Autodesk Inventor part; units mm, degrees
ref_plane "YZ Plane" through (0, 0, 0) normal (1, 0, 0) x (0, 1, 0)
ref_plane "XZ Plane" through (0, 0, 0) normal (0, 1, 0) x (-1, 0, 0)
ref_plane "XY Plane" through (0, 0, 0) normal (0, 0, 1) x (1, 0, 0)
sketch "Sketch1" plane through (0, 0, 0) normal (0, 1, 0) x (-1, 0, 0)
  circle A0 centre (0, 0) radius 75
  circle A1 centre (0, 0) radius 63.5
  line L0 (62, 12.5) -> (62, -12.5)
  line L1 (62, -12.5) -> (65, -12.5)
  line L2 (65, -12.5) -> (65, 12.5)
  line L3 (65, 12.5) -> (62, 12.5)
  line L4 (62, 12.5) -> (65, -12.5) construction
  line L5 (62, -12.5) -> (65, 12.5) construction
  line L6 (75, 0) -> (0, 0) construction
  line L7 (59.9334, 28.0933) -> (45.2388, 48.3188)
  line L8 (45.2388, 48.3188) -> (42.8117, 46.5554)
  line L9 (42.8117, 46.5554) -> (57.5064, 26.33)
  line L10 (57.5064, 26.33) -> (59.9334, 28.0933)
  line L11 (31.9743, 57.956) -> (8.1979, 65.6814)
  line L12 (8.1979, 65.6814) -> (7.2708, 62.8282)
  line L13 (7.2708, 62.8282) -> (31.0473, 55.1028)
  line L14 (31.0473, 55.1028) -> (31.9743, 57.956)
  line L15 (-8.1979, 65.6814) -> (-31.9743, 57.956)
  line L16 (-31.9743, 57.956) -> (-31.0473, 55.1028)
  line L17 (-31.0473, 55.1028) -> (-7.2708, 62.8282)
  line L18 (-7.2708, 62.8282) -> (-8.1979, 65.6814)
  line L19 (-45.2388, 48.3188) -> (-59.9334, 28.0933)
  line L20 (-59.9334, 28.0933) -> (-57.5064, 26.33)
  line L21 (-57.5064, 26.33) -> (-42.8117, 46.5554)
  line L22 (-42.8117, 46.5554) -> (-45.2388, 48.3188)
  line L23 (-65, 12.5) -> (-65, -12.5)
  line L24 (-65, -12.5) -> (-62, -12.5)
  line L25 (-62, -12.5) -> (-62, 12.5)
  line L26 (-62, 12.5) -> (-65, 12.5)
  line L27 (-59.9334, -28.0933) -> (-45.2388, -48.3188)
  line L28 (-45.2388, -48.3188) -> (-42.8117, -46.5554)
  line L29 (-42.8117, -46.5554) -> (-57.5064, -26.33)
  line L30 (-57.5064, -26.33) -> (-59.9334, -28.0933)
  line L31 (-31.9743, -57.956) -> (-8.1979, -65.6814)
  line L32 (-8.1979, -65.6814) -> (-7.2708, -62.8282)
  line L33 (-7.2708, -62.8282) -> (-31.0473, -55.1028)
  line L34 (-31.0473, -55.1028) -> (-31.9743, -57.956)
  line L35 (8.1979, -65.6814) -> (31.9743, -57.956)
  line L36 (31.9743, -57.956) -> (31.0473, -55.1028)
  line L37 (31.0473, -55.1028) -> (7.2708, -62.8282)
  line L38 (7.2708, -62.8282) -> (8.1979, -65.6814)
  line L39 (45.2388, -48.3188) -> (59.9334, -28.0933)
  line L40 (59.9334, -28.0933) -> (57.5064, -26.33)
  line L41 (57.5064, -26.33) -> (42.8117, -46.5554)
  line L42 (42.8117, -46.5554) -> (45.2388, -48.3188)
  circle A2 centre (75, 0) radius 2
  line L43 (74.8331, 5) -> (73.1411, 0.738)
  line L44 (73.1411, -0.738) -> (74.8331, -5)
  circle A3 centre (60.6763, 44.0839) radius 2
  line L45 (57.6024, 48.0309) -> (58.7386, 43.5883)
  line L46 (59.6062, 42.3942) -> (63.4802, 39.9407)
  circle A4 centre (23.1763, 71.3292) radius 2
  line L47 (18.3694, 72.7156) -> (21.9, 69.7894)
  line L48 (23.3037, 69.3333) -> (27.88, 69.6255)
  circle A5 centre (-23.1763, 71.3292) radius 2
  line L49 (-27.88, 69.6255) -> (-23.3037, 69.3333)
  line L50 (-21.9, 69.7894) -> (-18.3694, 72.7156)
  circle A6 centre (-60.6763, 44.0839) radius 2
  line L51 (-63.4802, 39.9407) -> (-59.6062, 42.3942)
  line L52 (-58.7386, 43.5883) -> (-57.6024, 48.0309)
  circle A7 centre (-75, 0) radius 2
  line L53 (-74.8331, -5) -> (-73.1411, -0.738)
  line L54 (-73.1411, 0.738) -> (-74.8331, 5)
  circle A8 centre (-60.6763, -44.0839) radius 2
  line L55 (-57.6024, -48.0309) -> (-58.7386, -43.5883)
  line L56 (-59.6062, -42.3942) -> (-63.4802, -39.9407)
  circle A9 centre (-23.1763, -71.3292) radius 2
  line L57 (-18.3694, -72.7156) -> (-21.9, -69.7894)
  line L58 (-23.3037, -69.3333) -> (-27.88, -69.6255)
  circle A10 centre (23.1763, -71.3292) radius 2
  line L59 (27.88, -69.6255) -> (23.3037, -69.3333)
  line L60 (21.9, -69.7894) -> (18.3694, -72.7156)
  circle A11 centre (60.6763, -44.0839) radius 2
  line L61 (63.4802, -39.9407) -> (59.6062, -42.3942)
  line L62 (58.7386, -43.5883) -> (57.6024, -48.0309)
  point P0 (63.5, 0)
  point P1 (63.5, 0)
  point P2 (62.2575, -12.5)
  point P3 (57.7147, -26.4813)
  point P4 (43.0201, -46.7068)
  point P5 (31.1268, -55.3477)
  point P6 (7.3504, -63.0731)
  point P7 (-7.3504, -63.0731)
  point P8 (-31.1268, -55.3477)
  point P9 (-43.0201, -46.7068)
  point P10 (-57.7147, -26.4813)
  point P11 (-62.2575, -12.5)
  point P12 (-62.2575, 12.5)
  point P13 (-57.7147, 26.4813)
  point P14 (-43.0201, 46.7068)
  point P15 (-31.1268, 55.3477)
  point P16 (-7.3504, 63.0731)
  point P17 (7.3504, 63.0731)
  point P18 (31.1268, 55.3477)
  point P19 (43.0201, 46.7068)
  point P20 (57.7147, 26.4813)
  point P21 (62.2575, 12.5)
  point P22 (65, 0)
  dimension "d1" = 127
  dimension "d2" = 25
  dimension "d3" = 3
  dimension "d6" = 360
  dimension "d11" = 4
  dimension "d12" = 10
  dimension "d13" = 5
  dimension "d15" = 10
  dimension "d16" = 150
  dimension "d19" = 360
extrude "Extrusion1" add sketch "Sketch1" along normal blind 3 contours L43 A2 L44 A0 L61 A11 L62 L59 A10 L60 L57 A9 L58 L55 A8 L56 L53 A7 L54 L51 A6 L52 L49 A5 L50 L47 A4 L48 L45 A3 L46
properties part number "lamina_rotor"
Geometry: final body of the model. Coordinates: model frame, mm. A direction names the side the tool comes from. Round coordinates to 2 decimals unless told otherwise and drop trailing zeros. Order: outer loops, then holes, each group sorted by start corner. A loop starts at its lowest first (then second) coordinate and runs counter-clockwise, first axis right, second up. Notation, with made-up numbers: (29.5, 69.5) -> (74.5, 69.5) arc R9 ccw to (74.5, 78.5) -> close; hole circle Ø3 at (-18, -30.75). An arc over 180 degrees is marked (long way). Use one line per item in the form item = value. Start each with the question number.
1. Cut plane B-B (z = 8). Return the cut outline in (x, y).
2. Reachability of faces 1 (the face through (60.424, 1.479, 19.524)), 2 (the face through (44.294, 1.479, 60.523)) from +Z, -Z, +X, -X, +Y, -Y: full face, straight path, thin tool, end or side. Return the list, or none.
3. Cut plane A-A (x = -11.5). Return the cut outline in (y, z).
4. Draft query along X for faces 3 (the face through (-43.87, 1.48, 60.83)), 4 (the face through (60.36, 1.48, -19.72)), 5 (the face through (39.2, 3, 50.3)). Return one class per face: pulls with the +X half, pulls with the -X half, needs draft (parallel to the pull), parting line crosses it, or undercut.
5. Pin query (flat end, axial travel): pin 1 Ø1.5 at (x, y) = (-41.5, 1.5) entering from +Z; pin 2 Ø0.8 at (x, y) = (64, 1.5) entering from -Z; pin 3 Ø1.5 at (x, y) = (-45, 0.5) entering from -Z. Return the tip coordinate at first contact, or that it passes through.
6. Line query: probe 1 along X at (y, z) = (1, 50); probe 2 along Z at (x, y) = (22, 2.55); probe 3 along Z at (x, y) = (-9, 0.45). Output: solid intervals per line, ascending.
Solution:
q1.outline = (-74.57, 0) -> (-65, 0) -> (-65, 3) -> (-74.57, 3) -> close; (65, 0) -> (74.57, 0) -> (74.57, 3) -> (65, 3) -> close
q2.face_1 = +Y, -Y
q2.face_2 = +Z, +X, +Y, -Y
q3.outline = (0, -74.11) -> (3, -74.11) -> (3, -64.61) -> (0, -64.61) -> close; (0, 64.61) -> (3, 64.61) -> (3, 74.11) -> (0, 74.11) -> close
q4.face_3 = pulls with the -X half
q4.face_4 = undercut
q4.face_5 = needs draft
q5.pin_1 = 62.96
q5.pin_2 = -39.75
q5.pin_3 = -60.56
q6.probe_1 = -55.9 to -39.14, 39.14 to 55.9
q6.probe_2 = -69.71 to -61.2, 61.2 to 69.71
q6.probe_3 = -74.46 to -65.42, 65.42 to 74.46
